```python
from build123d import *

# Parameters (mm, degrees)
SKETCH_W     = 24.7
SKETCH_H     = 16.9
PAD_DEPTH    = 1.5
SKETCH001_W  = 21.744
SKETCH001_H  = 10.864
PAD001_DEPTH = 1
SKETCH002_W  = 12
SKETCH002_H  = 0.5
PAD002_DEPTH = 1
SKETCH003_W  = 12
SKETCH003_H  = 0.1
PAD003_DEPTH = 2.7
PAD004_DEPTH = 0.1
FILLET_R     = 0.5
FILLET001_R  = 1
FILLET002_R  = 1


with BuildPart() as part:
    # Sketch → Pad (new body)
    with BuildSketch(Plane.XY):
        Rectangle(SKETCH_W, SKETCH_H)
    extrude(amount=PAD_DEPTH)

    # Sketch001 (on Face6 of Pad) → Pad001 (join)
    with BuildSketch(Plane.XY.offset(1.5)):
        with Locations((0, 1)):
            Rectangle(SKETCH001_W, SKETCH001_H)
        with BuildLine():
            ThreePointArc((-4.565, -6.012), (-5.065, -6.512), (-4.565, -7.012))
            Line((-4.565, -7.012), (4.565, -7.012))
            ThreePointArc((4.565, -7.012), (5.065, -6.512), (4.565, -6.012))
            Line((4.565, -6.012), (-4.565, -6.012))
        make_face()
    extrude(amount=-PAD001_DEPTH)

    # Sketch002 (on Face6 of Pad001) → Pad002 (join)
    with BuildSketch(Plane.XZ.offset(8.45)):
        with Locations((0, 1.25)):
            Rectangle(SKETCH002_W, SKETCH002_H)
    extrude(amount=PAD002_DEPTH)

    # Sketch003 (on Face11 of Pad002) → Pad003 (join)
    with BuildSketch(Plane(origin=(0, 0, 1), x_dir=(1, 0, 0), z_dir=(0, 0, -1))):
        with Locations((0, 9.4)):
            Rectangle(SKETCH003_W, SKETCH003_H)
    extrude(amount=PAD003_DEPTH)

    # Sketch004 (on Face18 of Pad003) → Pad004 (join)
    with BuildSketch(Plane(origin=(0, 0, -1.7), x_dir=(1, 0, 0), z_dir=(0, 0, -1))):
        Polygon((-6, 9.45), (-11, 3.25), (-11, -0.55), (11, -0.55), (11, 3.25), (6, 9.45), align=None)
    extrude(amount=PAD004_DEPTH)

    # Fillet
    fillet_edges = [part.edges().sort_by_distance(p)[0] for p in [
        (-11, 0.55, -1.75),
        (11, 0.55, -1.75),
    ]]
    fillet(fillet_edges, radius=FILLET_R)

    # Fillet001
    fillet001_edges = [part.edges().sort_by_distance(p)[0] for p in [
        (-11, -3.25, -1.75),
    ]]
    fillet(fillet001_edges, radius=FILLET001_R)

    # Fillet002
    fillet002_edges = [part.edges().sort_by_distance(p)[0] for p in [
        (11, -3.25, -1.75),
    ]]
    fillet(fillet002_edges, radius=FILLET002_R)


solid = part.part
```
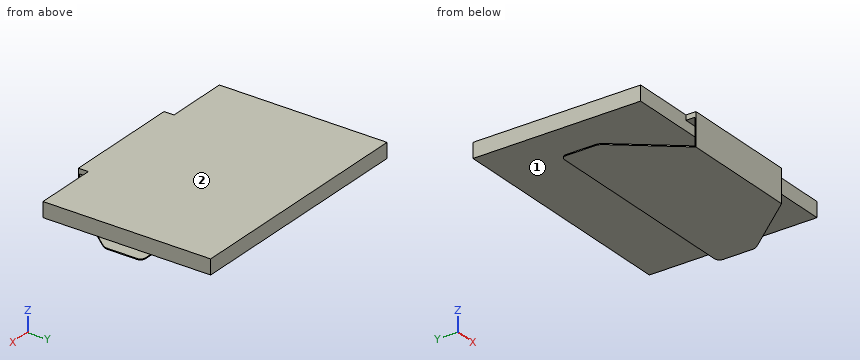
Build history of the part. All positions in model axes, mm. Face numbers are marked on the shaded views. A direction names the side the tool comes from. Round coordinates to 2 decimals unless told otherwise and drop trailing zeros. Order: outer loops, then holes, each group sorted by start corner. A loop starts at its lowest first (then second) coordinate and runs counter-clockwise, first axis right, second up. Notation, with made-up numbers: (76, 73.5) -> (119, 73.5) arc R30 cw to (119, 96.5) -> close; hole circle Ø7 at (38, 65.25). An arc over 180 degrees is marked (long way). Answer in a Markdown table with one row per item.
1) Wall check: L1, parallel to Y at x = 8, z = 1.2; L2, parallel to Z at x = 0, y = 1.25. Give the ranges that are in metal, low to high.
Values:
| item | result |
|---|---|
| L1 | -8.45 to 8.45 |
| L2 | 0 to 1.5 |
2) Band-saw the part on B-B on x = 7. Give the cut face in (y, z).
Values:
| item | result |
|---|---|
| outline | (-8.45, 0) -> (8.45, 0) -> (8.45, 1.5) -> (-8.45, 1.5) -> close; (-8.21, -1.8) -> (0.55, -1.8) -> (0.55, -1.7) -> (-8.21, -1.7) -> close |
3) Band-saw the part on A-A on y = -1.5. Give the cut face in (x, z), and give its area (4 significant figures).
Values:
| item | result |
|---|---|
| outline | (-12.35, 0) -> (12.35, 0) -> (12.35, 1.5) -> (-12.35, 1.5) -> close; (-11, -1.8) -> (11, -1.8) -> (11, -1.7) -> (-11, -1.7) -> close |
| area | 39.25 mm2 |
4) Band-saw the part on C-C on x = 0.75. Give the cut face in (y, z).
Values:
| item | result |
|---|---|
| outline | (-9.45, -1.8) -> (0.55, -1.8) -> (0.55, -1.7) -> (-9.35, -1.7) -> (-9.35, 1) -> (-8.45, 1) -> (-8.45, 0) -> (8.45, 0) -> (8.45, 1.5) -> (-9.45, 1.5) -> close |
5) Band-saw the part on D-D on z = -1.4. Give the cut face in (x, y).
Values:
| item | result |
|---|---|
| outline | (-6, -9.45) -> (6, -9.45) -> (6, -9.35) -> (-6, -9.35) -> close |
6) Which spindle directions (+Z, -Z, +X, -X, +Y, -Y) get a long thin tool onto all of the face, cutting with end or side? Do the marked faces 1 and 2. Say none if no direction does.
Values:
| item | result |
|---|---|
| face 1 | +X, -X, +Y |
| face 2 | +Z, +X, -X, +Y, -Y |
